```python
from build123d import *

# Parameters (mm, degrees)
BOSS_EXTRUDE1_DEPTH            = 20
SKETCH2_W                      = 20
SKETCH2_H                      = 23.5
BOSS_EXTRUDE2_DEPTH            = 4.5
CUT_EXTRUDE1_DEPTH             = 15
SKETCH4_W                      = 20
SKETCH4_H                      = 28
BOSS_EXTRUDE3_DEPTH            = 4.5
SKETCH5_W                      = 8
SKETCH5_H                      = 2
BOSS_EXTRUDE4_DEPTH            = 1
SKETCH6_W                      = 8
SKETCH6_H                      = 2
BOSS_EXTRUDE5_DEPTH            = 1
SKETCH7_W                      = 8
SKETCH7_H                      = 2
BOSS_EXTRUDE6_DEPTH            = 1
SKETCH8_W                      = 8
SKETCH8_H                      = 2
BOSS_EXTRUDE7_DEPTH            = 1
F_6_3_6_3_DIAMETER_HOLE1_D     = 6.3
F_6_3_6_3_DIAMETER_HOLE1_DEPTH = 28
F_6_3_6_3_DIAMETER_HOLE2_D     = 6.3
F_6_3_6_3_DIAMETER_HOLE2_DEPTH = 5.5
FILLET1_R                      = 0.3
FILLET2_START                  = -11
FILLET2_DEPTH                  = 22


with BuildPart() as part:
    # Sketch1 → Boss-Extrude1 (new body)
    with BuildSketch(Plane(origin=(-10, 0, 0), x_dir=(0, -1, 0), z_dir=(-1, 0, 0))):
        with BuildLine():
            Line((-28, 4.5), (-4.5, 4.5))
            Line((-4.5, 4.5), (-4.5, 28))
            Line((-4.5, 28), (-4.792893219, 27.707106781))
            add(Edge.make_bspline(
                [(-4.792893219, 27.707106781), (-12.430964406, 20.069035594), (-20.069035594, 12.430964406), (-27.707106781, 4.792893219)],
                knots=[0, 0, 0, 0, 1, 1, 1, 1], degree=3))
            Line((-27.707106781, 4.792893219), (-28, 4.5))
        make_face()
    extrude(amount=-BOSS_EXTRUDE1_DEPTH)

    # Sketch2 → Boss-Extrude2 (add)
    with BuildSketch(Plane.XZ.offset(-4.5)):
        with Locations((0, 16.25)):
            Rectangle(SKETCH2_W, SKETCH2_H)
    extrude(amount=BOSS_EXTRUDE2_DEPTH)

    # Sketch3 → Cut-Extrude1 (cut)
    with BuildSketch(Plane(origin=(-7.5, 0, 0), x_dir=(0, -1, 0), z_dir=(-1, 0, 0))):
        with BuildLine():
            Line((-4.5, 4.5), (-4.5, 28))
            Line((-4.5, 28), (-4.792893219, 27.707106781))
            add(Edge.make_bspline(
                [(-4.792893219, 27.707106781), (-12.430964406, 20.069035594), (-20.069035594, 12.430964406), (-27.707106781, 4.792893219)],
                knots=[0, 0, 0, 0, 1, 1, 1, 1], degree=3))
            Line((-27.707106781, 4.792893219), (-28, 4.5))
            Line((-28, 4.5), (-4.5, 4.5))
        make_face()
    extrude(amount=-CUT_EXTRUDE1_DEPTH, mode=Mode.SUBTRACT)

    # Sketch4 → Boss-Extrude3 (add)
    with BuildSketch(Plane(origin=(0, 0, 4.5), x_dir=(-1, 0, 0), z_dir=(0, 0, -1))):
        with Locations((0, 14)):
            Rectangle(SKETCH4_W, SKETCH4_H)
    extrude(amount=BOSS_EXTRUDE3_DEPTH)

    # Sketch5 → Boss-Extrude4 (add)
    with BuildSketch(Plane.XZ):
        with Locations((0, 24.5)):
            Rectangle(SKETCH5_W, SKETCH5_H)
    extrude(amount=BOSS_EXTRUDE4_DEPTH)

    # Sketch6 → Boss-Extrude5 (add)
    with BuildSketch(Plane.XZ):
        with Locations((0, 5)):
            Rectangle(SKETCH6_W, SKETCH6_H)
    extrude(amount=BOSS_EXTRUDE5_DEPTH)

    # Sketch7 → Boss-Extrude6 (add)
    with BuildSketch(Plane(origin=(0, 0, 0), x_dir=(-1, 0, 0), z_dir=(0, 0, -1))):
        with Locations((0, 5)):
            Rectangle(SKETCH7_W, SKETCH7_H)
    extrude(amount=BOSS_EXTRUDE6_DEPTH)

    # Sketch8 → Boss-Extrude7 (add)
    with BuildSketch(Plane(origin=(0, 0, 0), x_dir=(-1, 0, 0), z_dir=(0, 0, -1))):
        with Locations((0, 24.5)):
            Rectangle(SKETCH8_W, SKETCH8_H)
    extrude(amount=BOSS_EXTRUDE7_DEPTH)

    # Ø6.3 (6.3) Diameter Hole1
    with Locations(Plane(origin=(0, 0, 0), x_dir=(-1, 0, 0), z_dir=(0, 0, -1))):
        with Locations((0, 20)):
            Hole(F_6_3_6_3_DIAMETER_HOLE1_D / 2, depth=F_6_3_6_3_DIAMETER_HOLE1_DEPTH)

    # Ø6.3 (6.3) Diameter Hole2
    with Locations(Plane(origin=(0, 4.5, 0), x_dir=(1, 0, 0), z_dir=(0, 1, 0))):
        with Locations((0, -20)):
            Hole(F_6_3_6_3_DIAMETER_HOLE2_D / 2, depth=F_6_3_6_3_DIAMETER_HOLE2_DEPTH)

    # Fillet1
    fillet1_edges = [part.edges().sort_by_distance(p)[0] for p in [
        (-4, 23.5, -0.5),
        (-4, 25.5, -0.5),
        (4, 25.5, -0.5),
        (4, 23.5, -0.5),
        (4, -0.5, 25.5),
        (-4, -0.5, 25.5),
        (-4, -0.5, 23.5),
        (4, -0.5, 23.5),
        (4, -0.5, 6),
        (-4, -0.5, 6),
        (-4, -0.5, 4),
        (4, -0.5, 4),
        (-4, 4, -0.5),
        (-4, 6, -0.5),
        (4, 6, -0.5),
        (4, 4, -0.5),
    ]]
    fillet(fillet1_edges, radius=FILLET1_R)

    # Fillet2: read off the stored shape, not the designer's step
    # Fillet2 outline → Fillet2 (cut)
    with BuildSketch(Plane.YZ.offset(FILLET2_START)):
        with BuildLine():
            Line((28, 4.085786438), (28, 4.5))
            Line((28, 4.5), (27.707106781, 4.792893219))
            ThreePointArc((27.707106781, 4.792893219), (27.923879533, 4.46846987), (28, 4.085786438))
        make_face()
        with BuildLine():
            Line((4.792893219, 27.707106781), (4.5, 28))
            Line((4.5, 28), (4.085786438, 28))
            ThreePointArc((4.085786438, 28), (4.46846987, 27.923879533), (4.792893219, 27.707106781))
        make_face()
    extrude(amount=FILLET2_DEPTH, mode=Mode.SUBTRACT)


solid = part.part
```
Model file for the job. Use its own axes, mm. A direction names the side the tool comes from. Give positions to 0.01 mm unless a question says otherwise; leave off trailing zeros. Loops run counter-clockwise (first coordinate to the right, second up) from the corner with the lowest first, then second, coordinate; pieces in that order, holes last. Notation, with made-up numbers: (21.25, 33) -> (57.25, 33) arc R18 ccw to (57.25, 64) -> close; hole circle Ø2 at (-3.75, -14). An arc over 180 degrees is marked (long way). Write each question's results on one line, items separated by ' | '.
(1) Probe line 1 along X through (y, z) = (1.45, 20); line 2 along Y through (x, z) = (0, 2.4). List the from-to ranges inside material, lowest first.
Geometry results:
line 1: x = -10 to -3.15, 3.15 to 10 | line 2: y = 0 to 16.85, 23.15 to 28
(2) Cut at D-D on x = -4.5. List the corners of the cut face in (y, z).
Geometry results:
outline: (0, 0) -> (28, 0) -> (28, 4.09) arc R1 ccw to (27.91, 4.5) -> (4.5, 4.5) -> (4.5, 27.91) arc R1 ccw to (4.09, 28) -> (0, 28) -> close
(3) Cut at A-A on y = 20. List the corners of the cut face in (x, z).
Geometry results:
outline: (-10, 0) -> (-3.15, 0) -> (-3.15, 4.5) -> (-7.5, 4.5) -> (-7.5, 12.5) -> (-10, 12.5) -> close; (3.15, 0) -> (10, 0) -> (10, 12.5) -> (7.5, 12.5) -> (7.5, 4.5) -> (3.15, 4.5) -> close
(4) Cut at B-B on x = 0. Give the number of separate pieces and of enclosed holes in the cut face, and give its area (3 significant figures).
Geometry results:
separate pieces: 3 | enclosed holes: 0 | area: 183 mm²
(5) Pull direction Z, two halves, no side cores. Call faces 6 (the flat face through (-0.1, -0.5, 23.5)), 7 (the flat face through (0, 25, -1)), 8 (the flat face through (4, -0.5, 24.5)): released by +Z, released by -Z, zero draft, split by the parting line, or undercut.
Geometry results:
face 6: undercut | face 7: released by -Z | face 8: zero draft
(6) Tool access for faces 1 (the flat face through (-4, -0.5, 24.5)), 2 (the flat face through (4, 5, -0.5)), 3 (the flat face through (0.1, 23.5, -0.5)), 4 (the flat face through (7.5, 11, 11)), 5 (the flat face through (-0.1, -0.5, 6)): list every direction of +Z, -Z, +X, -X, +Y, -Y with a clear straight run to the whole face (end or side of a thin tool).
Geometry results:
face 1: +Z, -Z, -X, -Y | face 2: -Z, +X, +Y, -Y | face 3: -Z, +X, -X | face 4: +Z, +Y | face 5: +X, -X, -Y
(7) Flat gauge pins, fed straight in: pin 1 Ø0.8 at (y, z) = (-0.5, 5) entering from +X; pin 2 Ø8 at (x, z) = (-5, 7) entering from -Y; pin 3 Ø0.8 at (x, z) = (1.5, -0.5) entering from -Y; pin 4 Ø1 at (y, z) = (24.5, 11) entering from +X. Where does each tip first touch, or does it go through?
Geometry results:
pin 1: stops at x = 4 | pin 2: stops at y = -1 | pin 3: stops at y = 4 | pin 4: passes through
